Part model, mm, in its own coordinate system. Coordinates: 2 decimals unless noted, no trailing zeros. Loops run counter-clockwise (first coordinate to the right, second up) from the corner with the lowest first, then second, coordinate; pieces in that order, holes last. Notation, with made-up numbers: (-0.5, -10.5) -> (58.5, -10.5) arc R24 ccw to (58.5, 18.5) -> close; hole circle Ø2 at (30.25, -13.5). An arc over 180 degrees is marked (long way). Use one line per item in the form item = value. Start each with the question number.
(1) Mould opens along Z. For faces 1 (the cylindrical face through (-19.44, -9.86, 15.72)), 2 (the cylindrical face through (41.27, -9.86, -36.91)), 3 (the cylindrical face through (65.7, -9.9, 15.8)) say: +Z half, -Z half, draft (parallel to the pull), parting line (faces both ways), or undercut.
(2) Band-saw the part on A-A on z = -26. Give the cut face in (x, y), then the cut area to 3 significant figures.
(3) Band-saw the part on B-B on x = 52.5. Give the cut face in (y, z).
(4) Band-saw the part on D-D on x = -11.5. Give the cut face in (y, z), then the cut area to 3 significant figures.
(5) Pin check, flat tips, straight feed: P1, Ø4, axis at y = -12, z = -32.5, coming from the -X side; P2, Ø2, axis at x = 19.5, y = -9, coming from the -Z side; P3, Ø4, axis at x = 46.5, y = -6, coming from the +Z side. Stop position of each tip, or through.
(6) Band-saw the part on C-C on y = -13.25. Give the cut face in (x, z).
(7) Drill centre lines: L1, parallel to Z at x = 52.5, y = -5.75; L2, parallel to Z at x = 51, y = -7; L3, parallel to X at y = -0.75, z = 34.5. Where is each one in solid material? Low to high. Write a range as [from, to].
```python
from build123d import *

# Parameters (mm, degrees)
F0_R     = 10
F1_DEPTH = 20


with BuildPart() as f1:
    # F0 (on Front) → F1 (new body)
    with BuildSketch(Plane.XZ):
        with BuildLine():
            ThreePointArc((37.554206, 44.103474), (22.067235, 29.538399), (1.304766, 24.965929))
            ThreePointArc((1.304766, 24.965929), (-19.647756, 15.458515), (-23.957871, -7.142857))
            ThreePointArc((-23.957871, -7.142857), (-11.587381, -29.540201), (8.989835, -44.747049))
            ThreePointArc((8.989835, -44.747049), (17.576496, -47.837133), (26.532468, -49.589262))
            ThreePointArc((26.532468, -49.589262), (41.367793, -36.63373), (37.904534, -17.244596))
            ThreePointArc((37.904534, -17.244596), (36.990811, -9.071889), (44.120823, -4.974213))
            ThreePointArc((44.120823, -4.974213), (51.030762, -3.734261), (56.619703, 0.514089))
            ThreePointArc((56.619703, 0.514089), (65.792763, 16.032989), (69.941986, 33.576228))
            ThreePointArc((69.941986, 33.576228), (57.909572, 51.642912), (37.554206, 44.103474))
        make_face()
        Circle(F0_R, mode=Mode.SUBTRACT)
        with Locations((22.5, -30)):
            Circle(F0_R, mode=Mode.SUBTRACT)
        with Locations((52.5, 35)):
            Circle(F0_R, mode=Mode.SUBTRACT)
    extrude(amount=F1_DEPTH)


solid = f1.part
```
A:
q1.face_1 = parting line
q1.face_2 = undercut
q1.face_3 = -Z half
q2.outline = (-14.46, -20) -> (13.33, -20) -> (13.33, 0) -> (-14.46, 0) -> close; (31.67, -20) -> (42.1, -20) -> (42.1, 0) -> (31.67, 0) -> close
q2.area = 764 mm²
q3.outline = (-20, -2.99) -> (0, -2.99) -> (0, 25) -> (-20, 25) -> close; (-20, 45) -> (0, 45) -> (0, 52.5) -> (-20, 52.5) -> close
q4.outline = (-20, -29.64) -> (0, -29.64) -> (0, 22.2) -> (-20, 22.2) -> close
q4.area = 1,040 mm²
q5.P1 = -10.73
q5.P2 = -48.57
q5.P3 = 52.04
q6.outline = (-23.96, -7.14) arc R60 ccw to (8.99, -44.75) arc R60 ccw to (26.53, -49.59) arc R20 ccw to (37.9, -17.24) arc R7.5 cw to (44.12, -4.97) arc R15 ccw to (56.62, 0.51) arc R60 ccw to (69.94, 33.58) arc R17.5 ccw to (37.55, 44.1) arc R40 cw to (1.3, 24.97) arc R25 ccw to start; hole circle Ø20 at (0, 0); hole circle Ø20 at (22.5, -30); hole circle Ø20 at (52.5, 35)
q7.L1 = [-2.99, 25], [45, 52.5]
q7.L2 = [-3.75, 25.11], [44.89, 52.44]
q7.L3 = [29.38, 42.51], [62.49, 69.99]
